Verification items for the finished model (mm, model axes). Give positions to 0.01 mm unless a question says otherwise; leave off trailing zeros. Write each loop counter-clockwise with the first axis right and the second up, starting at its lowest first coordinate (ties: lowest second). Pieces come first, ordered by that corner, then holes.
Autodesk Inventor part; units mm, degrees
ref_plane "YZ Plane" through (0, 0, 0) normal (1, 0, 0) x (0, 1, 0)
ref_plane "XZ Plane" through (0, 0, 0) normal (0, 1, 0) x (-1, 0, 0)
ref_plane "XY Plane" through (0, 0, 0) normal (0, 0, 1) x (1, 0, 0)
sketch "Boceto1" plane through (0, 0, 0) normal (0, 0, 1) x (1, 0, 0)
  line L0 (0, 82.4534) -> (0, -82.4534) construction
  line L1 (-81.8976, 0) -> (81.8976, 0) construction
  line L2 (55, 49) -> (55, 24)
  arc A0 (55, 24) -> (55, 20) centre (55, 22) ccw
  line L3 (55, 20) -> (59, 20)
  line L4 (59, 20) -> (59, -20)
  line L5 (59, -20) -> (55, -20)
  arc A1 (55, -20) -> (55, -24) centre (55, -22) ccw
  line L6 (55, -24) -> (55, -49)
  line L7 (-55, 49) -> (-55, 24)
  arc A2 (-55, 20) -> (-55, 24) centre (-55, 22) ccw
  line L8 (-55, 20) -> (-59, 20)
  line L9 (-59, 20) -> (-59, -20)
  line L10 (-59, -20) -> (-55, -20)
  arc A3 (-55, -24) -> (-55, -20) centre (-55, -22) ccw
  line L11 (-55, -24) -> (-55, -49)
  line L12 (-49, 55) -> (-24, 55)
  line L13 (24, 55) -> (49, 55)
  line L14 (-49, -55) -> (-24, -55)
  line L15 (24, -55) -> (49, -55)
  arc A4 (-24, 55) -> (-20, 55) centre (-22, 55) ccw
  line L16 (-20, 55) -> (-20, 59)
  line L17 (-20, 59) -> (20, 59)
  line L18 (20, 59) -> (20, 55)
  arc A5 (20, 55) -> (24, 55) centre (22, 55) ccw
  arc A6 (-20, -55) -> (-24, -55) centre (-22, -55) ccw
  line L19 (-20, -55) -> (-20, -59)
  line L20 (-20, -59) -> (20, -59)
  line L21 (20, -59) -> (20, -55)
  arc A7 (24, -55) -> (20, -55) centre (22, -55) ccw
  line L22 (-55, 49) -> (-49, 55)
  line L23 (55, 49) -> (49, 55)
  line L24 (55, -49) -> (49, -55)
  line L25 (-49, -55) -> (-55, -49)
  line L26 (-40, 30) -> (-40, -30)
  arc A8 (-40, -30) -> (-30, -40) centre (-30, -30) ccw
  line L27 (-30, -40) -> (30, -40)
  arc A9 (30, -40) -> (40, -30) centre (30, -30) ccw
  line L28 (40, -30) -> (40, 30)
  arc A10 (40, 30) -> (30, 40) centre (30, 30) ccw
  line L29 (30, 40) -> (-30, 40)
  arc A11 (-30, 40) -> (-40, 30) centre (-30, 30) ccw
  point P0 (0, 0)
  point P1 (0, 0)
  point P2 (55, 55)
  point P3 (55, -55)
  point P4 (-55, 55)
  point P5 (-55, -55)
  point P6 (55, -55)
  point P7 (-59, 0)
  point P8 (55, -55)
  point P9 (-40, 0)
  point P10 (0, 40)
  dimension "d0" = 110
  dimension "d1" = 40
  dimension "d2" = 2
  dimension "d3" = 110
  dimension "d7" = 4
  dimension "d8" = 6
  dimension "d9" = 6
  dimension "d10" = 6
  dimension "d11" = 6
  dimension "d12" = 6
  dimension "d13" = 6
  dimension "d14" = 6
  dimension "d15" = 6
  dimension "d16" = 15
  dimension "d17" = 10
extrude "Extrusión1" add sketch "Boceto1" along normal mid plane 4
properties part number "refuerzo interior"
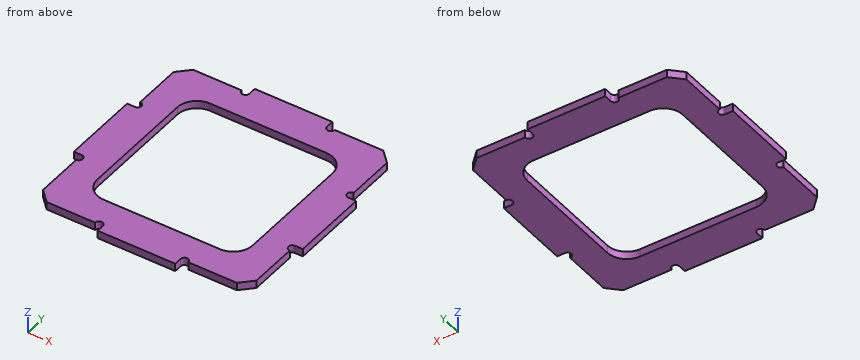
Item 1: Sectioned sample at A-A on x = 36. Record the cut outline in (y, z), then the cut area to 3 significant figures.
Answer key:
outline: (-55, -2) - (-38, -2) - (-38, 2) - (-55, 2) - close; (38, -2) - (55, -2) - (55, 2) - (38, 2) - close
area: 136 mm2
Item 2: Scan lines: line 1 along Y through (x, z) = (-1.5, 1.8); line 2 along X through (y, z) = (-24.5, -0.9). Record each from-to range of solid material in increasing order.
Answer key:
line 1: y = -59 to -40, 40 to 59
line 2: x = -55 to -40, 40 to 55
Item 3: Sectioned sample at C-C on y = 41.5. Record the cut outline in (x, z), then the cut area to 3 significant figures.
Answer key:
outline: (-55, -2) - (55, -2) - (55, 2) - (-55, 2) - close
area: 440 mm2
Item 4: Depth check by flat-ended pin: pin 1 (1.2 mm diameter, centred on x = -36, z = 0.5, fed in from +Y); pin 2 (12 mm diameter, centred on x = -19, y = -28.5, fed in from +Z); pin 3 (2 mm diameter, centred on y = -57.5, z = 0, fed in from +X); pin 4 (2 mm diameter, centred on y = -57, z = -1, fed in from -X). Enter the tip coordinate at first touch or a pass-through.
Answer key:
pin 1: stops at y = 55
pin 2: passes through
pin 3: stops at x = 20
pin 4: stops at x = -20
Item 5: Sectioned sample at B-B on y = 22. Record the cut outline in (x, z).
Answer key:
outline: (-53, -2) - (-40, -2) - (-40, 2) - (-53, 2) - close; (40, -2) - (53, -2) - (53, 2) - (40, 2) - close
